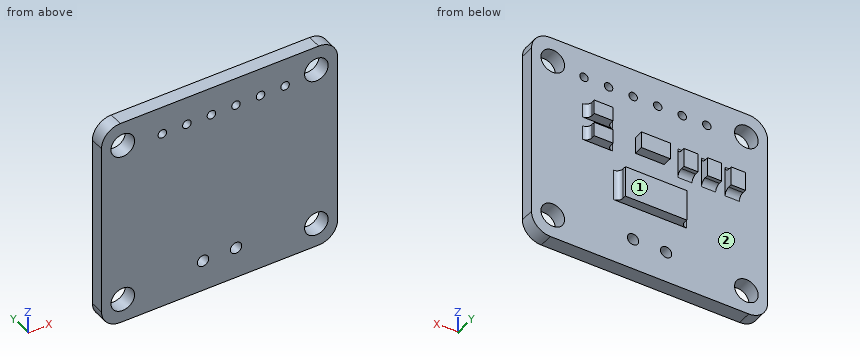
Autodesk Fusion 360 part; units mm, degrees
sketch "Sketch1" plane through (0, 0, 0) normal (0, 1, 0) x (1, 0, 0)
  line L0 (0, 0) -> (25, 0)
  line L1 (25, 0) -> (25, 22.3)
  line L2 (25, 22.3) -> (0, 22.3)
  line L3 (0, 22.3) -> (0, 0)
  dimension "d1" = 25
  dimension "d2" = 22.3
extrude "Extrude1" add sketch "Sketch1" along normal blind 1.5
fillet "Fillet1" radius 2 4 edges at (25, 0.75, 0) (25, 0.75, -22.3) (0, 0.75, -22.3) (0, 0.75, 0)
sketch "Sketch2" plane through (0, 1.5, 0) normal (0, 1, 0) x (-1, 0, 0)
  arc A0 (0, -2) -> (-2, 0) centre (-2, -2) ccw
  line L0 (-2, 0) -> (-23, 0)
  arc A1 (-23, 0) -> (-25, -2) centre (-23, -2) ccw
  line L1 (-25, -2) -> (-25, -20.3)
  arc A2 (-25, -20.3) -> (-23, -22.3) centre (-23, -20.3) ccw
  line L2 (-23, -22.3) -> (-2, -22.3)
  arc A3 (-2, -22.3) -> (0, -20.3) centre (-2, -20.3) ccw
  line L3 (0, -20.3) -> (0, -2)
  line L4 (0, 0) -> (-2.25, 0)
  line L5 (-2.25, 0) -> (-2.2498, -2.55)
  circle A4 centre (-2.2498, -2.55) radius 1.25
  line L6 (-2.2498, -2.55) -> (-2.2499, -1.275)
  line L7 (-2.2498, -2.55) -> (-2.2498, -19.8)
  circle A5 centre (-2.2498, -19.8) radius 1.25
  line L8 (0, 0) -> (-6.5, 0)
  line L9 (-6.5, 0) -> (-6.5, -0.4982)
  circle A6 centre (-6.44, -2.9975) radius 0.45
  line L10 (-6.44, -2.9975) -> (-9.04, -2.9948)
  circle A7 centre (-9.04, -2.9948) radius 0.45
  line L11 (-9.04, -2.9948) -> (-11.64, -2.9944)
  circle A8 centre (-11.64, -2.9944) radius 0.45
  line L12 (0, 0) -> (-10.75, 0)
  line L13 (-10.75, 0) -> (-10.75, -19)
  circle A9 centre (-10.75, -19) radius 0.6
  line L14 (-9.2, -15.4) -> (-15.7, -15.4)
  line L15 (-15.7, -15.4) -> (-15.7, -12.1)
  line L16 (-15.7, -12.1) -> (-9.2, -12.1)
  line L17 (-9.2, -12.1) -> (-9.2, -15.4)
  line L18 (-3, -9.5) -> (-4.5, -9.5)
  line L19 (-4.5, -9.5) -> (-4.5, -7.5)
  line L20 (-4.5, -7.5) -> (-3, -7.5)
  line L21 (-3, -7.5) -> (-3, -9.5)
  line L22 (-5.5, -9.5) -> (-7, -9.5)
  line L23 (-7, -9.5) -> (-7, -7.5)
  line L24 (-7, -7.5) -> (-5.5, -7.5)
  line L25 (-5.5, -7.5) -> (-5.5, -9.5)
  line L26 (-8, -9.5) -> (-9.5, -9.5)
  line L27 (-9.5, -9.5) -> (-9.5, -7.5)
  line L28 (-9.5, -7.5) -> (-8, -7.5)
  line L29 (-8, -7.5) -> (-8, -9.5)
  line L30 (-14, -7.5) -> (-10.9513, -7.5)
  line L31 (-10.9513, -7.5) -> (-10.9513, -9.2569)
  line L32 (-10.9513, -9.2569) -> (-14, -9.2569)
  line L33 (-14, -9.2569) -> (-14, -7.5)
  line L34 (-17, -10) -> (-19, -10)
  line L35 (-19, -10) -> (-19, -8.5)
  line L36 (-19, -8.5) -> (-17, -8.5)
  line L37 (-17, -8.5) -> (-17, -10)
  line L38 (-17, -7.5) -> (-19, -7.5)
  line L39 (-19, -7.5) -> (-19, -6)
  line L40 (-19, -6) -> (-17, -6)
  line L41 (-17, -6) -> (-17, -7.5)
  line L42 (-11.64, -2.9944) -> (-14.24, -2.9944)
  line L43 (-14.24, -2.9944) -> (-16.84, -2.9944)
  line L44 (-16.84, -2.9944) -> (-19.44, -2.9944)
  circle A10 centre (-14.24, -2.9944) radius 0.45
  circle A11 centre (-16.84, -2.9944) radius 0.45
  circle A12 centre (-19.44, -2.9944) radius 0.45
  dimension "d6" = 2.25
  dimension "d7" = 2.55
  dimension "d8" = 2.5
  dimension "d9" = 17.25
  dimension "d10" = 2.5
  dimension "d11" = 6.5
  dimension "d12" = 2.5
  dimension "d13" = 0.9
  dimension "d14" = 6.5
  dimension "d15" = 2.6
  dimension "d16" = 0.9
  dimension "d17" = 2.6
  dimension "d18" = 0.9
  dimension "d22" = 10.75
  dimension "d23" = 19
  dimension "d24" = 1.2
  dimension "d28" = 2.6
  dimension "d29" = 2.6
  dimension "d30" = 2.6
  dimension "d31" = 0.9
  dimension "d32" = 0.9
  dimension "d33" = 0.9
extrude "Extrude2" cut sketch "Sketch2" against normal blind 5 contours A5 | L5 A4 L6 L7 | L5 A4 L6 L7 | A9
ref_plane "WorkPlane1" through (12.5, 0.75, -11.15) normal (-1, 0, 0) x (0, 0, 1)
mirror "Mirror1" about plane through (12.5, 0.75, -11.15) normal (-1, 0, 0) of "Extrude2"
extrude "Extrude3" add sketch "Sketch2" along normal blind 1 contours L13 L14 L16 L17 | L13 L14 L15 L16 | L18 L19 L20 L21 | L22 L23 L24 L25 | L26 L27 L28 L29 | L30 L31 L32 L33 | L34 L35 L36 L37 | L38 L39 L40 L41
fillet "Fillet2" radius 0.6 12 edges at (9.2, 1.5, -13.75) (15.7, 1.5, -13.75) (8.75, 1.5, -7.5) (8.75, 1.5, -9.5) (6.25, 1.5, -7.5) (6.25, 1.5, -9.5) (3.75, 1.5, -9.5) (3.75, 1.5, -7.5) (19, 1.5, -9.25) (17, 1.5, -9.25) (17, 1.5, -6.75) (19, 1.5, -6.75)
extrude "Extrude4" cut sketch "Sketch2" against normal blind 4 contours A6 | L10 A7 L11 | L10 A7 L11 | A12 | L43 L44 A11 | L43 L44 A11 | L42 L43 A10 | L42 L43 A10 | L11 A8 L42 | L11 A8 L42
scale "Maßstab1" factor 0.9 about (3.4998, 1.5, -19.8) bodies 1
Geometry check sheet. Reference: the model listing, model coordinates, mm. Face numbers are marked on the shaded views. A direction names the side the tool comes from. Round coordinates to 2 decimals unless told otherwise and drop trailing zeros. Order: outer loops, then holes, each group sorted by start corner. A loop starts at its lowest first (then second) coordinate and runs counter-clockwise, first axis right, second up. Notation, with made-up numbers: M -31,64 L 8,64 A25 ccw 8,99 Z; hole C 26.5,88.5 d6. An arc over 180 degrees is marked long. Answer in a Markdown table with one row per item.
(1) Go/stop test with flat-tipped pins: P1, Ø0.7, axis at x = 12.5, y = 2, coming from the +Z side; P2, Ø0.6, axis at x = 13.17, z = -19.08, coming from the +Y side (3 decimals); P3, Ø6, axis at x = 18, z = -16.5, coming from the +Y side; P4, Ø3, axis at x = 2.37, z = -19.8, coming from the -Y side. Record where each tip stops, or that it passes through.
Responses:
| item | result |
|---|---|
| P1 | stops at z = -8.73 |
| P2 | passes through |
| P3 | stops at y = 1.5 |
| P4 | stops at y = 0.15 |
(2) Sectioned sample at D-D, the plane x = 12. Record the cut outline in (y, z).
Responses:
| item | result |
|---|---|
| outline | M 0.15,-22.05 L 1.5,-22.05 L 1.5,-15.84 L 2.4,-15.84 L 2.4,-12.87 L 1.5,-12.87 L 1.5,-10.31 L 2.4,-10.31 L 2.4,-8.73 L 1.5,-8.73 L 1.5,-1.98 L 0.15,-1.98 Z |
(3) Sectioned sample at B-B, the plane x = 16.75. Record the cut outline in (y, z), and give its area (3 significant figures).
Responses:
| item | result |
|---|---|
| outline | M 0.15,-22.05 L 1.5,-22.05 L 1.5,-10.98 L 2.4,-10.98 L 2.4,-9.63 L 1.5,-9.63 L 1.5,-8.73 L 2.4,-8.73 L 2.4,-7.38 L 1.5,-7.38 L 1.5,-1.98 L 0.15,-1.98 Z |
| area | 29.5 mm² |
(4) Sectioned sample at C-C, the plane z = -19.08. Record the cut outline in (x, y).
Responses:
| item | result |
|---|---|
| outline | M 0.35,0.15 L 1.51,0.15 L 1.51,1.5 L 0.35,1.5 Z; M 3.24,0.15 L 9.48,0.15 L 9.48,1.5 L 3.24,1.5 Z; M 10.56,0.15 L 12.63,0.15 L 12.63,1.5 L 10.56,1.5 Z; M 13.71,0.15 L 19.96,0.15 L 19.96,1.5 L 13.71,1.5 Z; M 21.69,0.15 L 22.85,0.15 L 22.85,1.5 L 21.69,1.5 Z |
(5) Tool access check on the marked faces 1 and 2. Record the directions out of +Z, -Z, +X, -X, +Y, -Y that give a thin tool (end or side, any length) a straight path to the whole face; none if there is none.
Responses:
| item | result |
|---|---|
| face 1 | +Z, -Z, +X, -X, +Y |
| face 2 | +Y |
(6) Scan lines: probe 1 along X at (y, z) = (1.85, -9); probe 2 along X at (y, z) = (1.25, -19.8); probe 3 along Z at (x, y) = (16, 1.6). Record each from-to range of solid material in increasing order. Write a range as from..to.
Responses:
| item | result |
|---|---|
| probe 1 | x = 3.05..4.4, 5.3..6.65, 7.55..8.9, 10.21..12.95 |
| probe 2 | x = 0.35..1.25, 3.5..19.7, 21.95..22.85 |
| probe 3 | z = -10.98..-9.63, -8.73..-7.38 |
(7) Sectioned sample at A-A, the plane y = 1. State how many separate pieces and enclosed holes the cut face has, and give its area (3 significant figures).
Responses:
| item | result |
|---|---|
| separate pieces | 1 |
| enclosed holes | 12 |
| area | 428 mm² |
